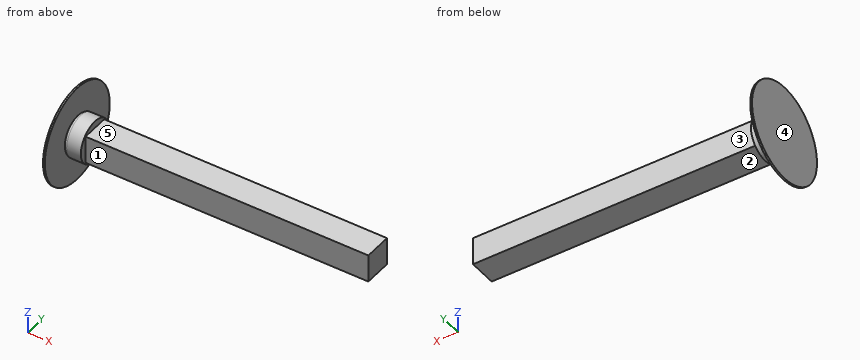
from build123d import *

# Parameters (mm, degrees)
F0_W     = 7.85
F0_H     = 7.85
F1_DEPTH = 85
F2_R     = 5.925
F3_DEPTH = 5
F4_R     = 1
F5_R     = 13.6615771023
F5_R_2   = 4.925
F6_DEPTH = 0.5


with BuildPart() as f1:
    # F0 (on Right) → F1 (new body)
    with BuildSketch(Plane.YZ):
        with Locations((16.0746219532, 0)):
            Rectangle(F0_W, F0_H)
    extrude(amount=F1_DEPTH)

    # F2 (on face) → F3 (join)
    with BuildSketch(Plane(origin=(0, 0, 0), x_dir=(0, -1, 0), z_dir=(-1, 0, 0))):
        with Locations((-16.0746219532, 0)):
            Circle(F2_R)
        Polygon((-19.9996219532, 3.925), (-16.0746219532, 3.925), (-12.1496219532, 3.925), (-12.1496219532, 0), (-12.1496219532, -3.925), (-16.0746219532, -3.925), (-19.9996219532, -3.925), (-19.9996219532, 0), align=None, mode=Mode.SUBTRACT)
    extrude(amount=-F3_DEPTH)

    # F4
    f4_edges = [f1.edges().sort_by_distance(p)[0] for p in [
        (0, 21.999622, 0),
    ]]
    fillet(f4_edges, radius=F4_R)

    # F5 (on face) → F6 (join)
    with BuildSketch(Plane(origin=(0, 0, 0), x_dir=(0, -1, 0), z_dir=(-1, 0, 0))):
        with Locations((-16.0746219532, 0)):
            Circle(F5_R)
        with Locations((-16.0746219532, 0)):
            Circle(F5_R_2, mode=Mode.SUBTRACT)
        with Locations((-16.0746219532, 0)):
            Circle(F5_R_2)
    extrude(amount=F6_DEPTH)


solid = f1.part
Verification items for the finished model (mm, model axes). Face numbers are marked on the shaded views. A direction names the side the tool comes from. Round coordinates to 2 decimals unless told otherwise and drop trailing zeros. Order: outer loops, then holes, each group sorted by start corner. A loop starts at its lowest first (then second) coordinate and runs counter-clockwise, first axis right, second up. Notation, with made-up numbers: (71, 71.25) -> (75, 71.25) arc R21 ccw to (75, 97.25) -> close; hole circle Ø4 at (87, 27.25). An arc over 180 degrees is marked (long way). Put each result on its own line as item: value.
1) Section check B-B (z = 0). Record the cut outline in (x, y).
Final values:
outline: (-0.5, 2.41) -> (0, 2.41) -> (0, 11.15) arc R1 ccw to (1, 10.15) -> (5, 10.15) -> (5, 12.15) -> (85, 12.15) -> (85, 20) -> (5, 20) -> (5, 22) -> (1, 22) arc R1 ccw to (0, 21) -> (0, 29.74) -> (-0.5, 29.74) -> close
2) Section check A-A (x = 62). Record the cut outline in (y, z) (3 decimals), then the cut area to 3 significant figures.
Final values:
outline: (12.15, -3.925) -> (20, -3.925) -> (20, 3.925) -> (12.15, 3.925) -> close
area: 61.6 mm^2
3) Set-up check for the marked faces 1, 2, 3, 4 and 5: record each of +Z, -Z, +X, -X, +Y, -Y from which the full face is reachable in a straight line by a thin tool's end or side.
Final values:
face 1: +Z, -Z, +X, -Y
face 2: -Z, +X, +Y, -Y
face 3: +Z, -Z, +X, +Y
face 4: +Z, -Z, -X, +Y, -Y
face 5: +Z, +X, +Y, -Y
4) Section check C-C (y = 6.75). Record the cut outline in (x, z), then the cut area to 3 significant figures.
Final values:
outline: (-0.5, -9.98) -> (0, -9.98) -> (0, 9.98) -> (-0.5, 9.98) -> close
area: 9.98 mm^2
5) Material ranges on line 1 (Z direction, x = 63, y = 17.25) (3 decimals); line 2 (X direction, y = 5.25, z = -7.5); line 3 (Y direction, x = 67, z = 1.25), recorded low to high.
Final values:
line 1: z = -3.925 to 3.925
line 2: x = -0.5 to 0
line 3: y = 12.15 to 20
6) Depth check by flat-ended pin: pin 1 (1 mm diameter, centred on x = 66, y = 10, fed in from -Z); pin 2 (2.5 mm diameter, centred on x = 33, y = 15, fed in from +Z) (3 decimals); pin 3 (4 mm diameter, centred on y = 13, z = 6, fed in from +X); pin 4 (8.5 mm diameter, centred on x = 37, y = 15, fed in from -Z) (3 decimals). Enter the tip coordinate at first touch or a pass-through.
Final values:
pin 1: passes through
pin 2: stops at z = 3.925
pin 3: stops at x = 5
pin 4: stops at z = -3.925
